The listing builds one solid part. Answer for the finished solid, in the listing's coordinates (mm). A direction names the side the tool comes from. Give positions to 0.01 mm unless a question says otherwise; leave off trailing zeros. Order: outer loops, then holes, each group sorted by start corner. A loop starts at its lowest first (then second) coordinate and runs counter-clockwise, first axis right, second up. Notation, with made-up numbers: (45.5, 58) - (75.5, 58) arc R32 cw to (75.5, 89) - close; hole circle Ø3 at (74, 71). An arc over 180 degrees is marked (long way). Answer as CSV lines item,"result". Start each with the question number.
1. Consider line 1 along X through (y, z) = (13.75, 71); line 2 along Z through (x, y) = (2.1, 10); line 3 along X through (y, z) = (16.25, 60). Determine where each line is inside the solid, lowest interval first. Write a range as [from, to].
2. Section B-B on z = 10 is taken. Give the vertices of the cut face in (x, y).
3. Section A-A on y = 10 is taken. Give the vertices of the cut face in (x, z).
4. Which of the six approach directions +Z, -Z, +X, -X, +Y, -Y give full straight-line access (tool end or side, diameter ignored) to faces 4 (the flat face through (1, 10, 90)), 5 (the flat face through (-5, 14.3, 80.1))?
5. Section C-C on z = 80 is taken. Give the vertices of the cut face in (x, y), and give its area (3 significant figures).
6. A flat-ended cylindrical pin translates along its axis: pin 1 (1 mm diameter, centred on y = 17.5, z = 31.5, fed in from -X). Find the tip coordinate at first contact, or state that the pin passes through.
7. Section D-D on x = -6 is taken. Give the vertices of the cut face in (y, z), and give its area (3 significant figures).
8. Determine the mould class of faces 1 (the flat face through (1, 20, 44)), 2 (the cylindrical face through (-6.479, 8.698, 89.915)), 3 (the cylindrical face through (1.479, 7.236, 12.534)) for opening direction Z: +Z half, -Z half, draft (parallel to the pull), parting line (faces both ways), or undercut.
from build123d import *

# Parameters (mm, degrees)
F0_W     = 20
F0_H     = 90
F0_R     = 3.75
F0_R_2   = 4
F1_DEPTH = 3
F2_DEPTH = 5
F4_R     = 10
F5_DEPTH = 3


with BuildPart() as f1:
    # F0 (on Right) → F1 (new body)
    with BuildSketch(Plane.YZ):
        with Locations((10, 45)):
            Rectangle(F0_W, F0_H)
        with Locations((10, 10)):
            Circle(F0_R, mode=Mode.SUBTRACT)
        with Locations((10, 80)):
            Circle(F0_R_2, mode=Mode.SUBTRACT)
        with Locations((10, 80)):
            Circle(F0_R_2)
    extrude(amount=F1_DEPTH)

    # F0 (on Right) → F2 (join)
    with BuildSketch(Plane.YZ):
        with Locations((10, 80)):
            Circle(F0_R_2)
    extrude(amount=-F2_DEPTH)

    # F4 (on offset) → F5 (join)
    with BuildSketch(Plane.YZ.offset(-5)):
        with Locations((10, 80)):
            Circle(F4_R)
    extrude(amount=-F5_DEPTH)


solid = f1.part
Checks:
1,line 1,"x = [-8, -5], [0, 3]"
1,line 2,"z = [0, 6.25], [13.75, 90]"
1,line 3,"x = [0, 3]"
2,outline,"(0, 0) - (3, 0) - (3, 6.25) - (0, 6.25) - close; (0, 13.75) - (3, 13.75) - (3, 20) - (0, 20) - close"
3,outline,"(-8, 70) - (-5, 70) - (-5, 76) - (0, 76) - (0, 13.75) - (3, 13.75) - (3, 90) - (0, 90) - (0, 84) - (-5, 84) - (-5, 90) - (-8, 90) - close; (0, 0) - (3, 0) - (3, 6.25) - (0, 6.25) - close"
4,face 4,"+Z, +X, -X, +Y, -Y"
4,face 5,"none"
5,outline,"(-8, 0) - (-5, 0) - (-5, 6) - (0, 6) - (0, 0) - (3, 0) - (3, 20) - (0, 20) - (0, 14) - (-5, 14) - (-5, 20) - (-8, 20) - close"
5,area,"160 mm²"
6,pin 1,"stops at x = 0"
7,outline,"circle Ø20 at (10, 80)"
7,area,"314 mm²"
8,face 1,"draft"
8,face 2,"parting line"
8,face 3,"undercut"
